Autodesk Inventor part; units mm, degrees
ref_plane "YZ Plane" through (0, 0, 0) normal (1, 0, 0) x (0, 1, 0)
ref_plane "XZ Plane" through (0, 0, 0) normal (0, 1, 0) x (-1, 0, 0)
ref_plane "XY Plane" through (0, 0, 0) normal (0, 0, 1) x (1, 0, 0)
sketch "Sketch1" plane through (0, 0, 0) normal (0, 1, 0) x (-1, 0, 0)
  arc A0 (0, -4) -> (0, 4) centre (0, 0) ccw
  line L0 (0, 4) -> (0, -4) construction
  line L1 (0, 4) -> (0, 9)
  line L2 (0, -4) -> (0, -9)
  line L3 (0, 9) -> (0.5, 9)
  line L4 (0.5, 9) -> (0.5, 16)
  line L5 (0, -9) -> (0.5, -9)
  line L6 (0.5, -9) -> (0.5, -16)
  line L7 (0.5, 16) -> (5.5, 16)
  line L8 (0.5, -16) -> (5.5, -16)
  line L9 (5.5, 16) -> (5.5, 9)
  line L10 (5.5, -16) -> (5.5, -9)
  line L11 (8, 0) -> (8, -6) construction
  line L12 (8, 0) -> (8, 6) construction
  line L13 (8, 6) -> (8, -6)
  line L14 (5.5, 9) -> (8, 6)
  line L15 (5.5, -9) -> (8, -6)
  dimension "d0" = 8
  dimension "d1" = 8
  dimension "d2" = 5
  dimension "d3" = 5
  dimension "d4" = 0.5
  dimension "d5" = 7
  dimension "d6" = 7
  dimension "d8" = 5
  dimension "d9" = 5
  dimension "d10" = 0
  dimension "d11" = 7
  dimension "d12" = 7
  dimension "d13" = 6
  dimension "d14" = 6
  dimension "d15" = 8
  dimension "d17" = 140.194
extrude "Extrusion1" add sketch "Sketch1" along normal blind 16
sketch "Sketch2" plane through (-8, 0, -6) normal (-1, 0, 0) x (0, 0, 1)
  line L0 (15, 0) -> (22, 0)
  line L1 (22, 0) -> (22, 16)
  line L2 (15, 16) -> (22, 16)
  line L3 (15, 0) -> (15, 16)
  line L4 (0, 0) -> (12, 0)
  line L5 (12, 0) -> (12, 16)
  line L6 (0, 16) -> (12, 16)
  line L7 (0, 0) -> (0, 16)
  line L8 (-10, 0) -> (-3, 0)
  line L9 (-3, 0) -> (-3, 16)
  line L10 (-10, 16) -> (-3, 16)
  line L11 (-10, 0) -> (-10, 16)
  circle A0 centre (6, 8) radius 1.5
  line L12 (4, 16) -> (12, 16)
  line L13 (8, 16) -> (20.5, 16)
  line L14 (0, 16) -> (16, 16)
  line L15 (8, 16) -> (-4.5, 16)
  line L16 (-1.3536, 16) -> (-7.8536, 16)
  line L17 (6.1, 7.993) -> (18.6, 7.993) construction
  line L18 (16.8536, 0) -> (16.8536, 16) construction
  line L19 (18.6, 7.993) -> (18.6, 3.993) construction
  line L20 (18.6, 3.993) -> (18.6, 11.993) construction
  line L21 (6.1, 7.993) -> (-6.5036, 7.993) construction
  line L22 (-6.5036, 7.993) -> (-6.5036, 3.993) construction
  line L23 (-6.5036, 3.993) -> (-6.5036, 11.993) construction
  circle A1 centre (18.6, 3.993) radius 1.75
  circle A2 centre (18.6, 11.993) radius 1.75
  circle A3 centre (-6.5036, 3.993) radius 1.75
  circle A4 centre (-6.5036, 11.993) radius 1.75
  point P0 (6, 0)
  point P1 (8, 0)
  dimension "d22" = 3
  dimension "d38" = 12.5
  dimension "d39" = 12.5
  dimension "d40" = 4
  dimension "d41" = 8
  dimension "d42" = 3.5
  dimension "d43" = 3.5
  dimension "d44" = 3.5
  dimension "d45" = 3.5
  dimension "d46" = 3.6
  dimension "d47" = 90
  dimension "d48" = 90
  dimension "d49" = 90
  dimension "d50" = 90
  dimension "d51" = 5.1464
  dimension "d52" = 28.5036
  dimension "d53" = 8.007
  dimension "d54" = 0
  dimension "d55" = 0
  dimension "d56" = 1.5
  dimension "d57" = 0
  dimension "d58" = 16
  dimension "d59" = 6
  dimension "d60" = 10
  dimension "d61" = 14
  dimension "d62" = 16
  dimension "d63" = 15.9
  dimension "d64" = 16
  dimension "d65" = 8
  dimension "d66" = 22
  dimension "d67" = 23.3535
  dimension "d68" = 4.007
  dimension "d69" = 12.007
  dimension "d70" = 29.8535
extrude "Extrusion3" cut sketch "Sketch2" against normal through all contours A0
chamfer "Chamfer1" distance 1 angle 45 1 edges at (-8, 8, -1.5)
chamfer "Chamfer2" distance 0.4 angle 45 2 edges at (0, 8, 9) (0, 8, -9)
extrude "Extrusion5" cut sketch "Sketch2" against normal blind 15 contours A1 | A2 | A3 | A4
properties part number "reverse gear  upper base bearing holder 1"
The listing builds one solid part. Answer for the finished solid, in the listing's coordinates (mm). A direction names the side the tool comes from. Coordinates: 2 decimals unless noted, no trailing zeros. Loops run counter-clockwise (first coordinate to the right, second up) from the corner with the lowest first, then second, coordinate; pieces in that order, holes last.
1) Find section D-D on z = 12.6. Write down the section's boundary in (x, y), then the cut area to 3 significant figures.
2) A tool of negligible diameter and unlimited length cuts with its end or side. For faces 4 (the face through (-3.035, 10.285, -12.883)), 5 (the face through (-0.5, 8, -12)), 6 (the face through (-5.5, 8, -13)), 7 (the face through (-0.5, 8, 12)), from which of +Z, -Z, +X, -X, +Y, -Y can it reach the whole face along a straight path? Write none if from no direction.
3) Find section C-C on x = -2.5. Write down the section's boundary in (y, z), then the cut area to 3 significant figures.
4) Find section B-B on y = 8. Write down the section's boundary in (x, z), then the cut area to 3 significant figures.
5) Find the intervals of material crossed by L1, parallel to Y at x = -1.6, z = 12.6; L2, parallel to Z at x = -5, y = 3.25; L3, parallel to Y at x = -3.25, z = 12, in increasing order.
6) Determine the mould class of faces 1 (the face through (-6.732, 7.888, 7.521)), 2 (the face through (-5.5, 8, 13)), 3 (the face through (-3.035, 11.323, 14.217)) for opening direction Z: pulls with the +Z half, pulls with the -Z half, needs draft (parallel to the pull), parting line crosses it, or undercut.
7) Flat-ended cylindrical pins translate along their axes: pin 1 Ø5.5 at (y, z) = (11.993, 12.6) entering from +X; pin 2 Ø7.5 at (y, z) = (12, -13) entering from -X; pin 3 Ø4 at (y, z) = (8, 0) entering from +X. Find the tip coordinate at first contact, or state that the pin passes through.
8) Find section A-A on z = 0. Write down the section's boundary in (x, y), then the cut area to 3 significant figures.
Values:
1. outline: (-5.5, 0) - (-0.5, 0) - (-0.5, 2.24) - (-5.5, 2.24) - close; (-5.5, 5.74) - (-0.5, 5.74) - (-0.5, 10.24) - (-5.5, 10.24) - close; (-5.5, 13.74) - (-0.5, 13.74) - (-0.5, 16) - (-5.5, 16) - close
1. area: 45.0 mm2
2. face 4: +X, -X
2. face 5: -Z, +X, +Y, -Y
2. face 6: -Z, -X, +Y, -Y
2. face 7: +Z, +X, +Y, -Y
3. outline: (0, -16) - (16, -16) - (16, -3.12) - (0, -3.12) - close; (0, 3.12) - (16, 3.12) - (16, 16) - (0, 16) - close; hole circle Ø3.5 at (3.99, -12.5); hole circle Ø3.5 at (3.99, 12.6); hole circle Ø3.5 at (11.99, -12.5); hole circle Ø3.5 at (11.99, 12.6)
3. area: 374 mm2
4. outline: (-8, -6) - (-5.5, -9) - (-5.5, -16) - (-0.5, -16) - (-0.5, -9) - (-0.4, -9) - (0, -8.6) - (0, -4) arc R4 cw to (-3.71, -1.5) - (-7, -1.5) - (-8, -2.5) - close; (-8, 2.5) - (-7, 1.5) - (-3.71, 1.5) arc R4 cw to (0, 4) - (0, 8.6) - (-0.4, 9) - (-0.5, 9) - (-0.5, 16) - (-5.5, 16) - (-5.5, 9) - (-8, 6) - close
4. area: 168 mm2
5. L1: y = 0 to 2.24, 5.74 to 10.24, 13.74 to 16
5. L2: z = -16 to -14.09, -10.92 to 11.02, 14.18 to 16
5. L3: y = 0 to 2.35, 5.64 to 10.35, 13.64 to 16
6. face 1: pulls with the +Z half
6. face 2: needs draft
6. face 3: undercut
7. pin 1: stops at x = -0.5
7. pin 2: stops at x = -5.5
7. pin 3: stops at x = -3.46
8. outline: (-8, 0) - (-4, 0) - (-4, 6.5) - (-7, 6.5) - (-8, 5.5) - close; (-8, 10.5) - (-7, 9.5) - (-4, 9.5) - (-4, 16) - (-8, 16) - close
8. area: 51.0 mm2
